from build123d import *
from OCP.BRepFilletAPI import BRepFilletAPI_MakeFillet

# Parameters (mm, degrees)
SKETCH_1_R          = 1.35
EXTRUDE_1_DEPTH     = 3
EXTRUDE_2_DEPTH     = 3
CUT_EXTRUDE_1_DEPTH = 10
FILLET_1_R1         = 1
FILLET_1_R2         = 2
FILLET_1_R3         = 10
FILLET_2_R          = 1


with BuildPart() as part:
    # 草图1 → 凸台-拉伸1 (new body)
    with BuildSketch(Plane(origin=(0, 0, 0), x_dir=(1, 0, 0), z_dir=(0, 1, 0))):
        Polygon((0, 35), (20, 35), (20, 20), (85, 20), (85, 0), (0, 0), (0, 10), align=None)
        with Locations(Location((76.5, 3, 0), (0, 0, 270))):
            Circle(SKETCH_1_R, mode=Mode.SUBTRACT)
        with Locations(Location((76.5, 17, 0), (0, 0, 90))):
            Circle(SKETCH_1_R, mode=Mode.SUBTRACT)
        with Locations(Location((28.5, 17, 0), (0, 0, 270))):
            Circle(SKETCH_1_R, mode=Mode.SUBTRACT)
        with Locations(Location((28.5, 3, 0), (0, 0, 90))):
            Circle(SKETCH_1_R, mode=Mode.SUBTRACT)
        with Locations(Location((4, 10, 0), (0, 0, 270))):
            Circle(SKETCH_1_R, mode=Mode.SUBTRACT)
        with Locations(Location((4, 30, 0), (0, 0, 90))):
            Circle(SKETCH_1_R, mode=Mode.SUBTRACT)
        with Locations(Location((16, 30, 0), (0, 0, 270))):
            Circle(SKETCH_1_R, mode=Mode.SUBTRACT)
        with Locations(Location((16, 10, 0), (0, 0, 90))):
            Circle(SKETCH_1_R, mode=Mode.SUBTRACT)
    extrude(amount=EXTRUDE_1_DEPTH)

    # 草图3 → 凸台-拉伸2 (add)
    with BuildSketch(Plane.XZ):
        Polygon((20, -31.755784464), (20, -35), (56.44071813, -20), (48.55928187, -20), align=None)
    extrude(amount=-EXTRUDE_2_DEPTH)

    # 草图4 → 切除-拉伸1 (cut)
    with BuildSketch(Plane.XZ):
        Polygon((34.571447814, -3), (41.75, -8.432417871), (48.928552186, -3), align=None)
        Polygon((32.5, -4.567582129), (32.5, -15.432417871), (39.678552186, -10), align=None)
        Polygon((41.75, -11.567582129), (34.571447814, -17), (48.928552186, -17), align=None)
        Polygon((51, -4.567582129), (43.821447814, -10), (51, -15.432417871), align=None)
        Polygon((54, -15.432417871), (61.178552186, -10), (54, -4.567582129), align=None)
        Polygon((70.428552186, -3), (56.071447814, -3), (63.25, -8.432417871), align=None)
        Polygon((72.5, -4.567582129), (65.321447814, -10), (72.5, -15.432417871), align=None)
        Polygon((70.428552186, -17), (63.25, -11.567582129), (56.071447814, -17), align=None)
    extrude(amount=-CUT_EXTRUDE_1_DEPTH, mode=Mode.SUBTRACT)

    # 圆角1: one fillet with a radius per group of edges: ONE call of the kernel's fillet builder (fillet() takes one radius for all edges)
    fillet_1_edges_1 = [part.edges().sort_by_distance(p)[0] for p in [
        (48.55928187, 1.5, -20),
    ]]
    fillet_1_edges_2 = [part.edges().sort_by_distance(p)[0] for p in [
        (20, 1.5, -20),
        (20, 1.5, -31.755784464),
        (0, 1.5, -35),
        (0, 1.5, 0),
        (85, 1.5, 0),
        (85, 1.5, -20),
    ]]
    fillet_1_edges_3 = [part.edges().sort_by_distance(p)[0] for p in [
        (56.44071813, 1.5, -20),
        (20, 1.5, -35),
    ]]
    fillet_1 = BRepFilletAPI_MakeFillet(part.part.solid().wrapped)
    for e in fillet_1_edges_1:
        fillet_1.Add(FILLET_1_R1, e.wrapped)
    for e in fillet_1_edges_2:
        fillet_1.Add(FILLET_1_R2, e.wrapped)
    for e in fillet_1_edges_3:
        fillet_1.Add(FILLET_1_R3, e.wrapped)
    add(Compound.cast(fillet_1.Shape()), mode=Mode.REPLACE)

    # 圆角2
    fillet_2_edges = [part.edges().sort_by_distance(p)[0] for p in [
        (43.821447814, 1.5, -10),
        (51, 1.5, -4.567582129),
        (51, 1.5, -15.432417871),
        (39.678552186, 1.5, -10),
        (32.5, 1.5, -15.432417871),
        (32.5, 1.5, -4.567582129),
        (34.571447814, 1.5, -17),
        (41.75, 1.5, -11.567582129),
        (48.928552186, 1.5, -17),
        (70.428552186, 1.5, -17),
        (56.071447814, 1.5, -17),
        (63.25, 1.5, -11.567582129),
        (70.428552186, 1.5, -3),
        (63.25, 1.5, -8.432417871),
        (56.071447814, 1.5, -3),
        (72.5, 1.5, -15.432417871),
        (65.321447814, 1.5, -10),
        (72.5, 1.5, -4.567582129),
        (48.928552186, 1.5, -3),
        (41.75, 1.5, -8.432417871),
        (34.571447814, 1.5, -3),
        (54, 1.5, -15.432417871),
        (54, 1.5, -4.567582129),
        (61.178552186, 1.5, -10),
    ]]
    fillet(fillet_2_edges, radius=FILLET_2_R)


solid = part.part
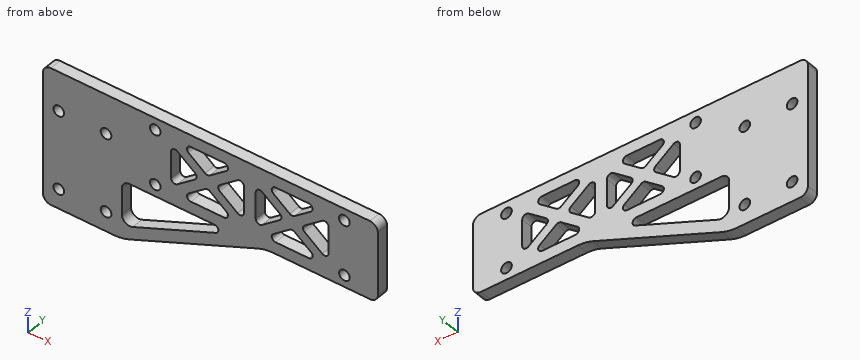
Source: CAD feature listing. Evaluate the final solid. Frame: model axes, mm. Coordinates: 2 decimals unless noted, no trailing zeros. Loops run counter-clockwise (first coordinate to the right, second up) from the corner with the lowest first, then second, coordinate; pieces in that order, holes last. Notation, with made-up numbers: (29, 24) - (52, 24) arc R10 ccw to (52, 36) - close; hole circle Ø8 at (64, 61.25). An arc over 180 degrees is marked (long way). One line per item, written item: value. Start each with the question number.
1. Section A-A (x = 76.5). Return the cut outline in (y, z), and give its area (3 significant figures).
2. Section C-C (y = 0.8). State how many separate pieces and enclosed holes the cut face has, and give its area (3 significant figures).
3. Ray query, L1, parallel to Z at x = 76.5, y = 1; L2, parallel to X at y = 0.8, z = -30; L3, parallel to Z at x = 65, y = 0.4. Return the intervals inside material, ascending.
4. Contact query for flat-ended pins moving along their axis: P1, Ø12, axis at x = 28, z = -12, coming from the -Y side; P2, Ø0.9, axis at y = 1, z = -26, coming from the +X side; P3, Ø1.5, axis at x = 62, y = 1.5, coming from the -Z side. Output: stop coordinate, or through.
5. Section B-B (z = -10). Return the cut outline in (x, y).
6. Section D-D (z = -27). Return the cut outline in (x, y), and give its area (3 significant figures).
Verdict:
1. outline: (0, -20) - (3, -20) - (3, -18.35) - (0, -18.35) - close; (0, -15.65) - (3, -15.65) - (3, -4.35) - (0, -4.35) - close; (0, -1.65) - (3, -1.65) - (3, 0) - (0, 0) - close
1. area: 43.8 mm2
2. separate pieces: 1
2. enclosed holes: 17
2. area: 1,770 mm2
3. L1: z = -20 to -18.35, -15.65 to -4.35, -1.65 to 0
3. L2: x = 0 to 2.65, 5.35 to 14.65, 17.35 to 20.42, 24.27 to 32.15
3. L3: z = -20 to -17, -12.89 to -7.11, -3 to 0
4. P1: stops at y = 0
4. P2: stops at x = 42.96
4. P3: stops at z = -20
5. outline: (0, 0) - (2.65, 0) - (2.65, 3) - (0, 3) - close; (5.35, 0) - (14.65, 0) - (14.65, 3) - (5.35, 3) - close; (17.35, 0) - (32.5, 0) - (32.5, 3) - (17.35, 3) - close; (39.02, 0) - (44.48, 0) - (44.48, 3) - (39.02, 3) - close; (51, 0) - (54, 0) - (54, 3) - (51, 3) - close; (60.52, 0) - (65.98, 0) - (65.98, 3) - (60.52, 3) - close; (72.5, 0) - (85, 0) - (85, 3) - (72.5, 3) - close
6. outline: (0, 0) - (20, 0) - (20, 3) - (0, 3) - close; (31.55, 0) - (39.44, 0) - (39.44, 3) - (31.55, 3) - close
6. area: 83.6 mm2
